Geometry: final body of the model. Coordinates: model frame, mm. Face numbers are marked on the shaded views. Coordinates: 2 decimals unless noted, no trailing zeros. Write each loop counter-clockwise with the first axis right and the second up, starting at its lowest first coordinate (ties: lowest second). Pieces come first, ordered by that corner, then holes. Notation, with made-up numbers: M 26,51.5 L 68,51.5 A21 cw 68,72.5 Z; hole C 24.25,-3 d11. An arc over 180 degrees is marked long. Write item = value, one per line. Start each with the question number.
Item 1: Section D-D on x = -36.5. Output: boundary loops of the cut face in (y, z), plus the area to 3 significant figures.
Item 2: Section C-C on x = 38.1. Output: boundary loops of the cut face in (y, z), plus the area to 3 significant figures.
Item 3: Ray query, L1, parallel to X at y = -6, z = 9.5; L2, parallel to Z at x = 38.1, y = -12.75; L3, parallel to X at y = -10.75, z = 5.5. Return the intervals inside material, ascending. Write a range as [from, to].
Item 4: First-contact query: pin 1 Ø1.8 at (y, z) = (-12.5, 41) entering from +X; pin 2 Ø5 at (x, z) = (-7.5, 41) entering from -Y (3 decimals); pin 3 Ø4 at (x, y) = (18.5, -8) entering from +Z. Flat tips, straight axial feed; report the tip coordinate or a pass-through.
Item 5: Pull-direction query (Z, two-part tool) for the marked faces 1, 2 and 3; classes: +Z half, -Z half, draft (parallel to the pull), parting line (faces both ways), or undercut.
Item 6: Section B-B on y = -12. Output: boundary loops of the cut face in (x, z).
Item 7: Section A-A on z = 0. Output: boundary loops of the cut face in (x, y).
from build123d import *

# Parameters (mm, degrees)
F0_W     = 76.2
F0_H     = 76.2
F0_R     = 12.7
F2_DEPTH = 18.796
F1_W     = 12.7
F1_H     = 6.35
F3_DEPTH = 44.196


with BuildPart() as f2:
    # F0 (on Front) → F2 (new body)
    with BuildSketch(Plane.XZ):
        with Locations((38.1, 0)):
            Rectangle(F0_W, F0_H)
        with Locations((38.1, 0)):
            Circle(F0_R, mode=Mode.SUBTRACT)
        with Locations((-38.1, 0)):
            Rectangle(F0_W, F0_H)
        with Locations((-38.1, 0)):
            Circle(F0_R, mode=Mode.SUBTRACT)
    extrude(amount=F2_DEPTH)

    # F1 (on Top) → F3 (join)
    with BuildSketch(Plane.XY):
        with Locations((-6.35, -12.7)):
            Rectangle(F1_W, F1_H)
    extrude(amount=F3_DEPTH)


solid = f2.part
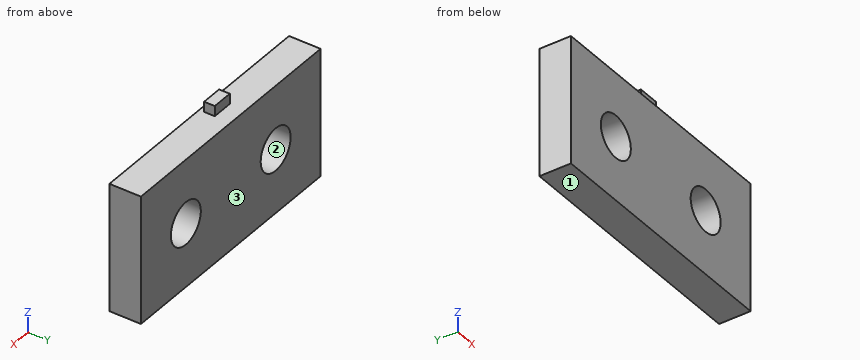
Responses:
q1.outline = M -18.8,-38.1 L 0,-38.1 L 0,-12.6 L -18.8,-12.6 Z; M -18.8,12.6 L 0,12.6 L 0,38.1 L -18.8,38.1 Z
q1.area = 959 mm²
q2.outline = M -18.8,-38.1 L 0,-38.1 L 0,-12.7 L -18.8,-12.7 Z; M -18.8,12.7 L 0,12.7 L 0,38.1 L -18.8,38.1 Z
q2.area = 955 mm²
q3.L1 = [-76.2, -46.53], [-29.67, 29.67], [46.53, 76.2]
q3.L2 = [-38.1, -12.7], [12.7, 38.1]
q3.L3 = [-76.2, -49.55], [-26.65, 26.65], [49.55, 76.2]
q4.pin_1 = 0
q4.pin_2 = -15.875
q4.pin_3 = 38.1
q5.face_1 = -Z half
q5.face_2 = undercut
q5.face_3 = draft
q6.outline = M -76.2,-38.1 L 76.2,-38.1 L 76.2,38.1 L 0,38.1 L 0,44.2 L -12.7,44.2 L -12.7,38.1 L -76.2,38.1 Z; hole C -38.1,0 d25.4; hole C 38.1,0 d25.4
q7.outline = M -76.2,-18.8 L -50.8,-18.8 L -50.8,0 L -76.2,0 Z; M -25.4,-18.8 L 25.4,-18.8 L 25.4,0 L -25.4,0 Z; M 50.8,-18.8 L 76.2,-18.8 L 76.2,0 L 50.8,0 Z
